Geometry check sheet. Reference: the model listing, model coordinates, mm. A direction names the side the tool comes from. Round coordinates to 2 decimals unless told otherwise and drop trailing zeros. Order: outer loops, then holes, each group sorted by start corner. A loop starts at its lowest first (then second) coordinate and runs counter-clockwise, first axis right, second up.
(1) Go/stop test with flat-tipped pins: pin 1 (4 mm diameter, centred on x = 6.5, z = 3, fed in from +Y); pin 2 (8 mm diameter, centred on y = 11, z = -1.5, fed in from +X); pin 3 (5 mm diameter, centred on x = 10.5, y = 14.5, fed in from -Z). Record where each tip stops, or that it passes through.
(2) Sectioned sample at B-B (x = 7.75). Record the boundary of the cut face in (y, z).
(3) Set-up check for faces 1 (the face through (9.307, 5.916, 3.693)), 2 (the face through (5, 0, 2.7)), 3 (the face through (7, 13, 5)): record each of +Z, -Z, +X, -X, +Y, -Y from which the full face is reachable in a straight line by a thin tool's end or side.
(4) Sectioned sample at C-C (y = 9.25). Record the boundary of the cut face in (x, z).
(5) Sectioned sample at A-A (z = 2.75). Record the boundary of the cut face in (x, y), plus the area to 3 significant figures.
(6) Release check for a two-part mould opening along Z. For faces 4 (the face through (-0.54, 12.32, -1.13)), 5 (the face through (8.53, 19.084, 0.955)), 6 (the face through (3, 25, 3)) record: +Z half, -Z half, draft (parallel to the pull), parting line (faces both ways), or undercut.
(7) Material ranges on line 1 along Z through (x, y) = (7, 13.25); line 2 along Z through (x, y) = (5.75, 3); line 3 along X through (y, z) = (22.5, 6), recorded low to high.
(8) Sectioned sample at D-D (z = 7.5). Record the boundary of the cut face in (x, y), plus the area to 3 significant figures.
Solid Edge part; units mm, degrees
sketch "Sketch1" plane through (0, 0, 0) normal (0, -1, 0) x (1, 0, 0)
  circle A0 centre (6.9977, 4.6504) radius 9.5
extrude "Protrusion1" add sketch "Sketch1" against normal blind 25
sketch "Sketch2" plane through (6.9977, 0, 4.6504) normal (0, -1, 0) x (1, 0, 0)
  circle A0 centre (0, 0) radius 2.5
extrude "VaciadoExtruido_1" cut sketch "Sketch2" against normal blind 12
sketch "Sketch3" plane through (6.9977, 25, 4.6504) normal (0, 1, 0) x (0, 0, -1)
  circle A0 centre (0, 0) radius 4
extrude "VaciadoExtruido_2" cut sketch "Sketch3" against normal blind 12
Answer below:
1. pin 1: stops at y = 13
1. pin 2: stops at x = 16.25
1. pin 3: stops at z = -4.8
2. outline: (0, -4.82) - (25, -4.82) - (25, 0.72) - (13, 0.72) - (13, 8.58) - (25, 8.58) - (25, 14.12) - (0, 14.12) - (0, 7.03) - (12, 7.03) - (12, 2.27) - (0, 2.27) - close
3. face 1: -Y
3. face 2: +Z, -Z, +X, -X, -Y
3. face 3: +Y
4. outline: circle Ø19 at (7, 4.65); hole circle Ø5 at (7, 4.65)
5. outline: (-2.31, 0) - (5.37, 0) - (5.37, 12) - (8.62, 12) - (8.62, 0) - (16.31, 0) - (16.31, 25) - (10.52, 25) - (10.52, 13) - (3.48, 13) - (3.48, 25) - (-2.31, 25) - close
5. area: 342 mm2
6. face 4: parting line
6. face 5: undercut
6. face 6: draft
7. line 1: z = -4.85 to 0.65, 8.65 to 14.15
7. line 2: z = -4.77 to 2.48, 6.82 to 14.07
7. line 3: x = -2.41 to 3.23, 10.76 to 16.4
8. outline: (-2.06, 0) - (16.06, 0) - (16.06, 25) - (9.8, 25) - (9.8, 13) - (4.19, 13) - (4.19, 25) - (-2.06, 25) - close
8. area: 386 mm2
